from build123d import *

# Parameters (mm, degrees)
BOSS_EXTRUDE1_DEPTH = 40


with BuildPart() as part:
    # Sketch1 → Boss-Extrude1 (new, symmetric)
    with BuildSketch(Plane(origin=(0, 0, 0), x_dir=(0, 0, -1), z_dir=(1, 0, 0))):
        with BuildLine():
            ThreePointArc((30, 0), (21.213203436, 21.213203436), (0, 30))
            Line((0, 30), (0, 20))
            ThreePointArc((0, 20), (14.142135624, 14.142135624), (20, 0))
            ThreePointArc((20, 0), (14.142135624, -14.142135624), (0, -20))
            Line((0, -20), (0, -30))
            ThreePointArc((0, -30), (21.213203436, -21.213203436), (30, 0))
        make_face()
        with BuildLine():
            Line((0, 20), (0, 30))
            ThreePointArc((0, 30), (-30, 0), (0, -30))
            Line((0, -30), (0, -20))
            ThreePointArc((0, -20), (-20, 0), (0, 20))
        make_face()
    extrude(amount=BOSS_EXTRUDE1_DEPTH, both=True)


solid = part.part
Model file for the job. Use its own axes, mm. Coordinates: 2 decimals unless noted, no trailing zeros. Order: outer loops, then holes, each group sorted by start corner. A loop starts at its lowest first (then second) coordinate and runs counter-clockwise, first axis right, second up. Notation, with made-up numbers: M 5,78 L 27,78 A20 ccw 27,99 Z; hole C 25.5,-36 d10. An arc over 180 degrees is marked long. Return JSON: item names as keys, results as strings.
1. Saw through at B-B (z = -11.5). Give the cut face in (x, y).
Ans:
{"outline": "M -40,-27.71 L 40,-27.71 L 40,-16.36 L -40,-16.36 Z; M -40,16.36 L 40,16.36 L 40,27.71 L -40,27.71 Z"}
2. Saw through at C-C (y = -7.5). Give the cut face in (x, z), and give its area (3 significant figures).
Ans:
{"outline": "M -40,-29.05 L 40,-29.05 L 40,-18.54 L -40,-18.54 Z; M -40,18.54 L 40,18.54 L 40,29.05 L -40,29.05 Z", "area": "1,680 mm^2"}
3. Saw through at D-D (y = -22.5). Give the cut face in (x, z), and give its area (3 significant figures).
Ans:
{"outline": "M -40,-19.84 L 40,-19.84 L 40,19.84 L -40,19.84 Z", "area": "3,170 mm^2"}
4. Flat gauge pins, fed straight in: pin 1 (6 mm diameter, centred on x = 2, z = 15.5, fed in from +Y); pin 2 (1 mm diameter, centred on x = 11, z = 2.5, fed in from +Y); pin 3 (6 mm diameter, centred on x = -1.5, y = -14, fed in from -Z). Where does each tip first touch, or does it go through?
Ans:
{"pin 1": "y = 27.27", "pin 2": "y = 29.93", "pin 3": "z = -27.91"}
5. Saw through at A-A (x = -10). Give the cut face in (y, z), and give its area (3 significant figures).
Ans:
{"outline": "C 0,0 d60; hole C 0,0 d40", "area": "1,570 mm^2"}
6. Drill centre lines: probe 1 along Z at (x, y) = (-32.5, -13.5); probe 2 along Y at (x, z) = (-21, 8); probe 3 along Z at (x, y) = (11, -5). Where is each one in solid material? Low to high.
Ans:
{"probe 1": "-26.79 to -14.76, 14.76 to 26.79", "probe 2": "-28.91 to -18.33, 18.33 to 28.91", "probe 3": "-29.58 to -19.36, 19.36 to 29.58"}
